```python
from build123d import *

# Parameters (mm, degrees)
SKETCH_1_R                = 3
EXTRUDE_1_DEPTH           = 15
DOME_1_FACE_RADIUS        = 3
DOME_1_HEIGHT             = 3
SKETCH_4_R                = 3.5
EXTRUDE_2_DEPTH           = 26
SKETCH_5_R                = 3.5
SKETCH_5_R_2              = 3
CUT_EXTRUDE_3_DEPTH       = 7
EXTRUDE_START             = -13
SKETCH_6_R                = 5.5
EXTRUDE_3_DEPTH           = 2.5
HOLE_WIZARD_4_0_4_1_D     = 4
HOLE_WIZARD_4_0_4_1_DEPTH = 7.5
HOLE_WIZARD_4_0_4_1_TIP   = 1.201721238
HOLE_WIZARD_3_0_3_1_D     = 3
HOLE_WIZARD_3_0_3_1_DEPTH = 9
HOLE_WIZARD_3_0_3_1_TIP   = 0.901290929
CUT_EXTRUDE_4_DEPTH       = 6.5
CUT_EXTRUDE_4_DEPTH_BACK  = 6.5


with BuildPart() as part:
    # Sketch 1 → Extrude 1 (new body)
    with BuildSketch(Plane.XY):
        Circle(SKETCH_1_R)
    extrude(amount=EXTRUDE_1_DEPTH)

    # Dome 1: a dome of height H over a round flat face of radius A is a cap of a sphere of radius (A * A + H * H) / (2 * H)
    dome_1_r = (DOME_1_FACE_RADIUS * DOME_1_FACE_RADIUS + DOME_1_HEIGHT * DOME_1_HEIGHT) / (2 * DOME_1_HEIGHT)
    dome_1_base = Plane((0, 0, 15), z_dir=(0, 0, 1))
    with Locations(dome_1_base.offset(DOME_1_HEIGHT - dome_1_r)):
        dome_1_ball = Sphere(dome_1_r, mode=Mode.PRIVATE)
    add(split(dome_1_ball, bisect_by=dome_1_base, keep=Keep.TOP, mode=Mode.PRIVATE))

    # Sketch 4 → Extrude 2 (add)
    with BuildSketch(Plane(origin=(0, 0, 0), x_dir=(-1, 0, 0), z_dir=(0, 0, -1))):
        Circle(SKETCH_4_R)
    extrude(amount=EXTRUDE_2_DEPTH)

    # Sketch 5 → Cut-Extrude 3 (cut)
    with BuildSketch(Plane(origin=(0, 0, -26), x_dir=(-1, 0, 0), z_dir=(0, 0, -1))):
        Circle(SKETCH_5_R)
        Circle(SKETCH_5_R_2, mode=Mode.SUBTRACT)
    extrude(amount=-CUT_EXTRUDE_3_DEPTH, mode=Mode.SUBTRACT)

    # Sketch 6 → Extrude 3 (add)
    with BuildSketch(Plane.XY.offset(EXTRUDE_START)):
        Circle(SKETCH_6_R)
    extrude(amount=-EXTRUDE_3_DEPTH)

    # Hole Wizard 4.0 _4_1
    with Locations(Plane(origin=(0, 0, -26), x_dir=(-1, 0, 0), z_dir=(0, 0, -1))):
        with Locations((0, 0)):
            Hole(HOLE_WIZARD_4_0_4_1_D / 2, depth=HOLE_WIZARD_4_0_4_1_DEPTH)
            with Locations((0, 0, -(HOLE_WIZARD_4_0_4_1_DEPTH + HOLE_WIZARD_4_0_4_1_TIP / 2))):  # 118° drill point
                Cone(0, HOLE_WIZARD_4_0_4_1_D / 2, HOLE_WIZARD_4_0_4_1_TIP, mode=Mode.SUBTRACT)

    # Hole Wizard 3.0 _3_1
    with Locations(Plane(origin=(-3, 0, -24), x_dir=(0, 0, -1), z_dir=(-1, 0, 0))):
        with Locations((0, 0)):
            Hole(HOLE_WIZARD_3_0_3_1_D / 2, depth=HOLE_WIZARD_3_0_3_1_DEPTH)
            with Locations((0, 0, -(HOLE_WIZARD_3_0_3_1_DEPTH + HOLE_WIZARD_3_0_3_1_TIP / 2))):  # 118° drill point
                Cone(0, HOLE_WIZARD_3_0_3_1_D / 2, HOLE_WIZARD_3_0_3_1_TIP, mode=Mode.SUBTRACT)

    # Sketch 12 → Cut-Extrude 4 (cut, two sides)
    with BuildSketch(Plane(origin=(0, 0, 0), x_dir=(1, 0, 0), z_dir=(0, 1, 0))) as cut_extrude_4_sk:
        Polygon((1.5, 26), (-3, 20), (-3, 26), align=None)
    extrude(amount=CUT_EXTRUDE_4_DEPTH, mode=Mode.SUBTRACT)
    extrude(cut_extrude_4_sk.sketch, amount=-CUT_EXTRUDE_4_DEPTH_BACK, mode=Mode.SUBTRACT)


solid = part.part
```
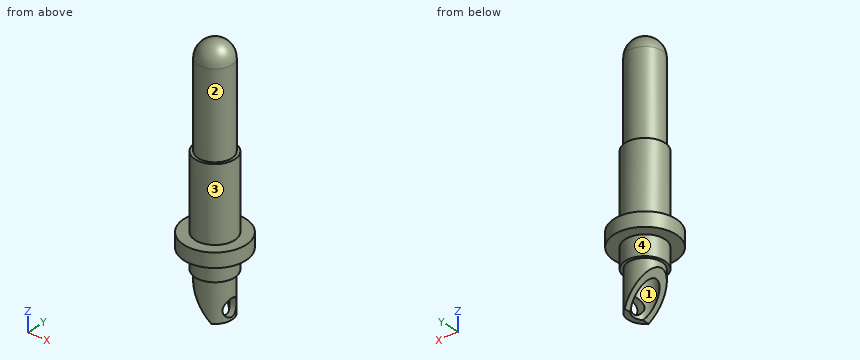
Geometry: final body of the model. Coordinates: model frame, mm. Face numbers are marked on the shaded views. A direction names the side the tool comes from. Round coordinates to 2 decimals unless told otherwise and drop trailing zeros. Write each loop counter-clockwise with the first axis right and the second up, starting at its lowest first coordinate (ties: lowest second). Pieces come first, ordered by that corner, then holes. Notation, with made-up numbers: (-40, 37.5) -> (-18, 37.5) arc R23 ccw to (-18, 59.5) -> close; hole circle Ø11 at (-2, 22). An arc over 180 degrees is marked (long way). Use CSV: the item, a comma, the result in double quotes. Start each with the question number.
Q1. Section D-D (y = -4.25). Return loops of the section in (x, z).
Q2. Pull-direction query (Y, two-part tool) for the marked faces 1 and 2; classes: pulls with the +Y half, pulls with the -Y half, needs draft (parallel to the pull), parting line crosses it, or undercut.
Q3. Section A-A (z = -24). Return loops of the section in (x, y), plus the area to 3 significant figures.
Q4. Reachability of the marked faces 3 and 4 from +Z, -Z, +X, -X, +Y, -Y: full face, straight path, thin tool, end or side. Return the list, or none.
Q5. First-contact query: pin 1 Ø1 at (x, z) = (3.5, -11) entering from +Y; pin 2 Ø2.5 at (x, y) = (0, 0) entering from -Z; pin 3 Ø2 at (x, y) = (-3.5, 1) entering from +Z. Flat tips, straight axial feed; report the tip coordinate or a pass-through.
Q6. Section C-C (z = -0.5). Return loops of the section in (x, y), plus the area to 3 significant figures.
Q7. Section B-B (x = -2.5). Return loops of the section in (y, z).
Q8. Line query: L1, parallel to Y at x = 0, z = -22.5; L2, parallel to Z at x = 3, y = 4.5; L3, parallel to Z at x = 2.5, y = 0. Output: solid intervals per line, ascending.
Result sheet:
1,outline,"(-3.49, -15.5) -> (3.49, -15.5) -> (3.49, -13) -> (-3.49, -13) -> close"
2,face 1,"undercut"
2,face 2,"parting line crosses it"
3,outline,"(0, -3) arc R3 ccw to (2.6, -1.5) -> (1.32, -1.5) arc R2 cw to (0, -2) -> close; (0, 2) arc R2 cw to (1.32, 1.5) -> (2.6, 1.5) arc R3 ccw to (0, 3) -> close"
3,area,"4.62 mm²"
4,face 3,"+Z"
4,face 4,"-Z"
5,pin 1,"y = 1.8"
5,pin 2,"z = -18.05"
5,pin 3,"z = 16.42"
6,outline,"circle Ø7 at (0, 0)"
6,area,"38.5 mm²"
7,outline,"(-4.9, -15.5) -> (-2.45, -15.5) -> (-2.45, -19) -> (-1.66, -19) -> (-1.66, -20.67) -> (1.66, -20.67) -> (1.66, -19) -> (2.45, -19) -> (2.45, -15.5) -> (4.9, -15.5) -> (4.9, -13) -> (2.45, -13) -> (2.45, 0) -> (1.66, 0) -> (1.66, 15) arc R1.66 ccw to (-1.66, 15) -> (-1.66, 0) -> (-2.45, 0) -> (-2.45, -13) -> (-4.9, -13) -> close"
8,L1,"-3 to -2, 2 to 3"
8,L2,"-15.5 to -13"
8,L3,"-26 to -25.5, -22.5 to 16.66"
